Read the model definition and answer for the solid it produces. Units are mm, in the model's axes. Face numbers are marked on the shaded views. Give positions to 0.01 mm unless a question says otherwise; leave off trailing zeros. Write each loop counter-clockwise with the first axis right and the second up, starting at its lowest first coordinate (ties: lowest second). Pieces come first, ordered by that corner, then holes. Notation, with made-up numbers: M 19,14.5 L 35,14.5 A24 cw 35,36.5 Z; hole C 80.25,-22.5 d7. An arc over 180 degrees is marked long. Put each result on its own line as item: value.
from build123d import *
from build123d.topology import SkipClean

# Parameters (mm, degrees)
SKETCH1_R               = 21
BOSS_EXTRUDE1_DEPTH     = 1.5
SKETCH2_R               = 2.65
CUT_EXTRUDE1_DEPTH      = 1.5
SKETCH5_W               = 10
SKETCH5_H               = 50
BOSS_EXTRUDE2_DEPTH     = 1.5
CIRPATTERN1_DEPTH       = 1.5
CUT_EXTRUDE4_REACH      = 56.252
SKETCH4_R               = 1.65
CUT_EXTRUDE5_REACH      = 56.314
SKETCH6_R               = 1.5
CUT_EXTRUDE6_DEPTH      = 55.251728083
CUT_EXTRUDE6_DEPTH_BACK = 55.251728083


# Read off the part's stored shape, not the designer's step: CirPattern1
with BuildPart() as part:
    # Sketch1 → Boss-Extrude1 (new, symmetric)
    with BuildSketch(Plane(origin=(0, 0, 0), x_dir=(1, 0, 0), z_dir=(0, 1, 0))):
        with Locations(Location((0, 0, 0), (0, 0, 270))):
            Circle(SKETCH1_R)
    extrude(amount=BOSS_EXTRUDE1_DEPTH, both=True)

    # Sketch2 → Cut-Extrude1 (cut)
    with BuildSketch(Plane(origin=(0, 1.5, 0), x_dir=(1, 0, 0), z_dir=(0, 1, 0))):
        with Locations((0, -15)):
            Circle(SKETCH2_R)
        with BuildLine():
            ThreePointArc((-2.65, -15), (0, -12.35), (2.65, -15))
            Line((2.65, -15), (4.067821782, -0.821782178))
            ThreePointArc((4.067821782, -0.821782178), (0, -4.15), (-4.067821782, -0.821782178))
            Line((-4.067821782, -0.821782178), (-2.65, -15))
        make_face()
        with BuildLine():
            ThreePointArc((-4.067821782, -0.821782178), (0, -4.15), (4.067821782, -0.821782178))
            Line((4.067821782, -0.821782178), (4.15, 0))
            ThreePointArc((4.15, 0), (0, 4.15), (-4.15, 0))
            Line((-4.15, 0), (-4.067821782, -0.821782178))
        make_face()
    cut_extrude1 = extrude(amount=-CUT_EXTRUDE1_DEPTH, mode=Mode.SUBTRACT)

    # Sketch5 → Boss-Extrude2 (add, symmetric)
    with BuildSketch(Plane(origin=(0, 0, 0), x_dir=(1, 0, 0), z_dir=(0, 1, 0))):
        with Locations((0, -25)):
            Rectangle(SKETCH5_W, SKETCH5_H)
    extrude(amount=BOSS_EXTRUDE2_DEPTH, both=True)

    # Mirror1: Cut-Extrude1 across plane
    with SkipClean():  # the faces are left unmerged after this step: merging them gives an invalid solid
        add(cut_extrude1.mirror(Plane.XY), mode=Mode.SUBTRACT)

    # CirPattern1 outline → CirPattern1 (cut)
    with BuildSketch(Plane(origin=(0, 0, 0), x_dir=(1, 0, 0), z_dir=(0, 1, 0))):
        with BuildLine():
            Line((3.772727273, -3.772727273), (15, -2.65))
            ThreePointArc((15, -2.65), (17.65, 0), (15, 2.65))
            Line((15, 2.65), (3.772727273, 3.772727273))
            Line((3.772727273, 3.772727273), (4.067821782, 0.821782178))
            ThreePointArc((4.067821782, 0.821782178), (0, -4.15), (-4.067821782, 0.821782178))
            Line((-4.067821782, 0.821782178), (-3.772727273, 3.772727273))
            Line((-3.772727273, 3.772727273), (-15, 2.65))
            ThreePointArc((-15, 2.65), (-17.65, 0), (-15, -2.65))
            Line((-15, -2.65), (-3.772727273, -3.772727273))
            Line((-3.772727273, -3.772727273), (-2.65, -15))
            ThreePointArc((-2.65, -15), (0, -17.65), (2.65, -15))
            Line((2.65, -15), (3.772727273, -3.772727273))
        make_face()
    extrude(amount=CIRPATTERN1_DEPTH, mode=Mode.SUBTRACT)

    # Sketch4 → Cut-Extrude4 (cut, up to next)
    with BuildSketch(Plane(origin=(0, 0, 0), x_dir=(1, 0, 0), z_dir=(0, 1, 0)), mode=Mode.PRIVATE) as cut_extrude4_sk1:
        with Locations(Location((0, 0, 0), (0, 0, 270))):
            Circle(SKETCH4_R)
    cut_extrude4_tool1 = extrude(cut_extrude4_sk1.sketch, amount=-CUT_EXTRUDE4_REACH, mode=Mode.PRIVATE) & part.part
    add(cut_extrude4_tool1.solids().sort_by_distance((0, 0, 0))[0], mode=Mode.SUBTRACT)

    # Sketch6 → Cut-Extrude5 (cut, up to next)
    with BuildSketch(Plane(origin=(0, 1.5, 0), x_dir=(1, 0, 0), z_dir=(0, 1, 0)), mode=Mode.PRIVATE) as cut_extrude5_sk1:
        with Locations(Location((0, -45.5, 0), (0, 0, 270))):
            Circle(SKETCH6_R)
    cut_extrude5_tool1 = extrude(cut_extrude5_sk1.sketch, amount=-CUT_EXTRUDE5_REACH, mode=Mode.PRIVATE) & part.part
    add(cut_extrude5_tool1.solids().sort_by_distance((0, 1.5, 45.5))[0], mode=Mode.SUBTRACT)

    # Sketch7 → Cut-Extrude6 (cut, two sides: drawn at the far end of the back side and taken through both)
    with BuildSketch(Plane(origin=(0, 0, 0), x_dir=(1, 0, 0), z_dir=(0, 1, 0)).offset(-CUT_EXTRUDE6_DEPTH_BACK)):
        with BuildLine():
            ThreePointArc((5, -20.396078054), (0, 21), (-5, -20.396078054))
            Line((-5, -20.396078054), (-5.519486194, -16.207382355))
            ThreePointArc((-5.519486194, -16.207382355), (-5.607043009, -15.695391034), (-5.647210443, -15.177522436))
            Line((-5.647210443, -15.177522436), (-6.513602442, -6.513602442))
            Line((-6.513602442, -6.513602442), (-15.177522436, -5.647210443))
            ThreePointArc((-15.177522436, -5.647210443), (-20.65, 0), (-15.177522436, 5.647210443))
            Line((-15.177522436, 5.647210443), (-6.513602442, 6.513602442))
            Line((-6.513602442, 6.513602442), (-5.647210443, 15.177522436))
            ThreePointArc((-5.647210443, 15.177522436), (0, 20.65), (5.647210443, 15.177522436))
            Line((5.647210443, 15.177522436), (6.513602442, 6.513602442))
            Line((6.513602442, 6.513602442), (15.177522436, 5.647210443))
            ThreePointArc((15.177522436, 5.647210443), (20.65, 0), (15.177522436, -5.647210443))
            Line((15.177522436, -5.647210443), (6.513602442, -6.513602442))
            Line((6.513602442, -6.513602442), (5.647210443, -15.177522436))
            ThreePointArc((5.647210443, -15.177522436), (5.607043009, -15.695391034), (5.519486194, -16.207382355))
            Line((5.519486194, -16.207382355), (5, -20.396078054))
        make_face()
    extrude(amount=CUT_EXTRUDE6_DEPTH + CUT_EXTRUDE6_DEPTH_BACK, mode=Mode.SUBTRACT)


solid = part.part
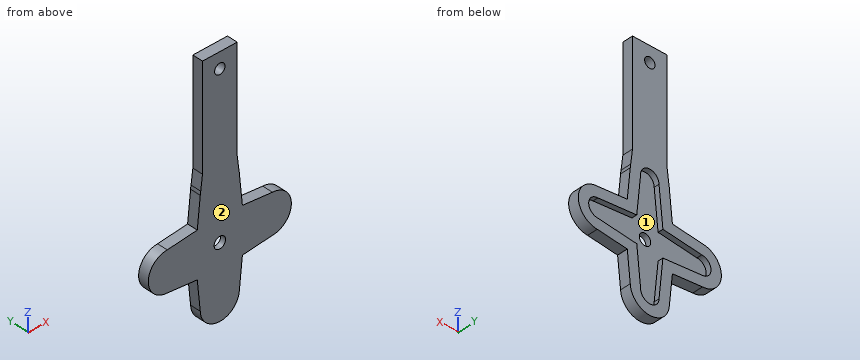
(1) For a pull along Z with two mould halves and no side action, classify the marked faces 1 and 2 as +Z half, -Z half, draft (parallel to the pull), parting line (faces both ways), or undercut.
Result:
face 1: undercut
face 2: draft
(2) Section B-B on x = 0 is taken. Determine the outline of the cut face in (y, z).
Result:
outline: M -1.5,-20.65 L 1.5,-20.65 L 1.5,-17.65 L 0,-17.65 L 0,-1.65 L -1.5,-1.65 Z; M -1.5,1.65 L 0,1.65 L 0,17.65 L 1.5,17.65 L 1.5,44 L -1.5,44 Z; M -1.5,47 L 1.5,47 L 1.5,50 L -1.5,50 Z
(3) Given pin 1 Ø1.5 at (y, z) = (0, 36) entering from +X; pin 2 Ø4 at (x, z) = (0, 0) entering from +Y, each flat-ended and moving along its own axis, determine where each tip first touches the part or whether it passes through.
Result:
pin 1: stops at x = 5
pin 2: stops at y = 0
(4) Straight lines are drawn through the part: line 1 along X through (y, z) = (0.6, 45.5); line 2 along X through (y, z) = (1.3, 35); line 3 along X through (y, z) = (-0.6, 0). For each, find the intervals that lie inside material, in ascending order. Write a range as from..to.
Result:
line 1: x = -5..-1.5, 1.5..5
line 2: x = -5..5
line 3: x = -20.65..-1.65, 1.65..20.65
(5) Section D-D on x = -13 is taken. Determine the outline of the cut face in (y, z), and give its area (3 significant figures).
Result:
outline: M -1.5,-5.86 L 1.5,-5.86 L 1.5,-2.85 L 0,-2.85 L 0,2.85 L 1.5,2.85 L 1.5,5.86 L -1.5,5.86 Z
area: 26.6 mm²
(6) Section A-A on z = 45.5 is taken. Determine the outline of the cut face in (x, y).
Result:
outline: M -5,-1.5 L -1.5,-1.5 L -1.5,1.5 L -5,1.5 Z; M 1.5,-1.5 L 5,-1.5 L 5,1.5 L 1.5,1.5 Z
